```python
from build123d import *

# Parameters (mm, degrees)
CUT_EXTRUDE1_DEPTH      = 11
CUT_EXTRUDE1_DEPTH_BACK = 11
SKETCH4_R               = 3.5
CUT_EXTRUDE2_DEPTH      = 15


with BuildPart() as part:
    # Sketch1 → Revolve1 (revolve)
    with BuildSketch(Plane.XY):
        with BuildLine():
            ThreePointArc((0, 20), (10, 10), (0, 0))
            Line((0, 0), (0, 20))
        make_face()
    revolve(axis=Axis((0, 0, 0), (0, 1, 0)))

    # Sketch3 → Cut-Extrude1 (cut, two sides)
    with BuildSketch(Plane.XY) as cut_extrude1_sk:
        Polygon((0, 17), (-8.309800503, 17), (-8.309800503, 20), (9.435235491, 20), (9.435235491, 17), align=None)
        Polygon((0, 0), (9.435235491, 0), (9.435235491, 3), (-8.578664685, 3), (-8.578664685, 0), align=None)
    extrude(amount=CUT_EXTRUDE1_DEPTH, mode=Mode.SUBTRACT)
    extrude(cut_extrude1_sk.sketch, amount=-CUT_EXTRUDE1_DEPTH_BACK, mode=Mode.SUBTRACT)

    # Sketch4 → Cut-Extrude2 (cut, through all)
    with BuildSketch(Plane(origin=(0, 17, 0), x_dir=(1, 0, 0), z_dir=(0, 1, 0))):
        Circle(SKETCH4_R)
    extrude(amount=-CUT_EXTRUDE2_DEPTH, mode=Mode.SUBTRACT)


solid = part.part
```
Can you work these out from the model? Positions are in its coordinate system, mm. Round coordinates to 2 decimals unless told otherwise and drop trailing zeros. Loops run counter-clockwise (first coordinate to the right, second up) from the corner with the lowest first, then second, coordinate; pieces in that order, holes last. Notation, with made-up numbers: M -12,-25.75 L 23,-25.75 A5 ccw 23,-21.75 Z; hole C -2,87.25 d10. An arc over 180 degrees is marked long. Answer as a JSON object with one key per item and string values. Group by question number.
Q1. Imagine slicing it at C-C, the plane y = 4.5. Please give me the cut outline in (x, z).
Q2. Please list where these lines run through material, in increasing order: L1, parallel to X at y = 8, z = 1.75; L2, parallel to X at y = 7.75, z = 0; L3, parallel to Z at x = 0, y = 6.
Q3. Imagine slicing it at A-A, the plane x = 0. Please give me the cut outline in (y, z).
Q4. Will these pins go through, and if not, where does the flat tip stop? pin 1 (4 mm diameter, centred on y = 4.5, z = -7.5, fed in from +X); pin 2 (5 mm diameter, centred on x = -1, y = 5.5, fed in from +Z); pin 3 (3 mm diameter, centred on x = 5, y = 14.5, fed in from +Z).
Q5. We'd pull the mould along Z, two halves only. Please class faces 1 (the cylindrical face through (3.233, 10.098, 1.341)), 2 (the flat face through (-1.7, 17, -3.3)): +Z half, -Z half, draft (parallel to the pull), parting line (faces both ways), or undercut.
Q6. Imagine slicing it at D-D, the plane z = 8. Please give me the cut outline in (x, y), then the cut area to 3 significant figures.
Q7. Imagine slicing it at B-B, the plane z = 1.25. Please give me the cut outline in (x, y).
Findings:
{
 "1": {"outline": "C 0,0 d16.7; hole C 0,0 d7"},
 "2": {"L1": "x = -9.64 to -3.03, 3.03 to 9.64", "L2": "x = -9.74 to -3.5, 3.5 to 9.74", "L3": "z = -9.17 to -3.5, 3.5 to 9.17"},
 "3": {"outline": "M 3,-7.14 A10 ccw 17,-7.14 L 17,-3.5 L 3,-3.5 Z; M 3,3.5 L 17,3.5 L 17,7.14 A10 ccw 3,7.14 Z"},
 "4": {"pin 1": "stops at x = 6.83", "pin 2": "stops at z = 9.77", "pin 3": "stops at z = 8.53"},
 "5": {"face 1": "undercut", "face 2": "draft"},
 "6": {"outline": "C 0,10 d12", "area": "113 mm2"},
 "7": {"outline": "M -7.03,3 L -3.27,3 L -3.27,17 L -7.03,17 A9.92 ccw Z; M 3.27,3 L 7.03,3 A9.92 ccw 7.03,17 L 3.27,17 Z"}
}
